from build123d import *

# Parameters (mm, degrees)
SKETCH1_R           = 1.5
SKETCH1_W           = 3
SKETCH1_H           = 7.2
SKETCH1_H_2         = 5
BOSS_EXTRUDE1_DEPTH = 3.5
FILLET1_R           = 2


with BuildPart() as part:
    # Sketch1 → Boss-Extrude1 (new body)
    with BuildSketch(Plane.XY):
        with BuildLine():
            Line((-6, 90), (-6, 5.139066063))
            ThreePointArc((-6, 5.139066063), (0, -7.9), (6, 5.139066063))
            Line((6, 5.139066063), (6, 90))
            ThreePointArc((6, 90), (0, 96), (-6, 90))
        make_face()
        Circle(SKETCH1_R, mode=Mode.SUBTRACT)
        with Locations((0, 60.876985236)):
            Circle(SKETCH1_R, mode=Mode.SUBTRACT)
        with Locations((0, 90)):
            Circle(SKETCH1_R, mode=Mode.SUBTRACT)
        with Locations((0, 25.976985236)):
            Rectangle(SKETCH1_W, SKETCH1_H, mode=Mode.SUBTRACT)
        with Locations((0, 79.876985236)):
            Rectangle(SKETCH1_W, SKETCH1_H_2, mode=Mode.SUBTRACT)
    extrude(amount=BOSS_EXTRUDE1_DEPTH)

    # Fillet1
    fillet1_edges = [part.edges().sort_by_distance(p)[0] for p in [
        (6, 5.139066063, 1.75),
        (-6, 5.139066063, 1.75),
    ]]
    fillet(fillet1_edges, radius=FILLET1_R)


solid = part.part
Design review of the part built by this model. Coordinates are the model's own, in mm. A direction names the side the tool comes from. Coordinates: 2 decimals unless noted, no trailing zeros. Write each loop counter-clockwise with the first axis right and the second up, starting at its lowest first coordinate (ties: lowest second). Pieces come first, ordered by that corner, then holes. Notation, with made-up numbers: (27.5, 74) - (55.5, 74) arc R16 ccw to (55.5, 95) - close; hole circle Ø9 at (29, -40). An arc over 180 degrees is marked (long way). Use one line per item in the form item = value.
Q1. Consider section C-C (z = 2.9). Write out the cut boundary in (x, y), plus the area to 3 significant figures.
Taken from the geometry:
outline = (-6.38, 4.65) arc R7.9 ccw (long way) to (6.38, 4.65) arc R2 cw to (6, 5.83) - (6, 90) arc R6 ccw to (-6, 90) - (-6, 5.83) arc R2 cw to start; hole circle Ø3 at (0, 0); hole (-1.5, 22.38) - (1.5, 22.38) - (1.5, 29.58) - (-1.5, 29.58) - close; hole circle Ø3 at (0, 60.88); hole (-1.5, 77.38) - (1.5, 77.38) - (1.5, 82.38) - (-1.5, 82.38) - close; hole circle Ø3 at (0, 90)
area = 1,190 mm^2
Q2. For probe 1 along Y at (x, z) = (0, 2.5); probe 2 along X at (y, z) = (90, 2.55); probe 3 along Y at (x, z) = (-1, 0.2), list the stretches that pass through material, from the lowest coordinate up.
Taken from the geometry:
probe_1 = -7.9 to -1.5, 1.5 to 22.38, 29.58 to 59.38, 62.38 to 77.38, 82.38 to 88.5, 91.5 to 96
probe_2 = -6 to -1.5, 1.5 to 6
probe_3 = -7.84 to -1.12, 1.12 to 22.38, 29.58 to 59.76, 62 to 77.38, 82.38 to 88.88, 91.12 to 95.92
Q3. Consider section B-B (x = 0). Write out the cut boundary in (y, z), plus the area to 3 significant figures.
Taken from the geometry:
outline = (-7.9, 0) - (-1.5, 0) - (-1.5, 3.5) - (-7.9, 3.5) - close; (1.5, 0) - (22.38, 0) - (22.38, 3.5) - (1.5, 3.5) - close; (29.58, 0) - (59.38, 0) - (59.38, 3.5) - (29.58, 3.5) - close; (62.38, 0) - (77.38, 0) - (77.38, 3.5) - (62.38, 3.5) - close; (82.38, 0) - (88.5, 0) - (88.5, 3.5) - (82.38, 3.5) - close; (91.5, 0) - (96, 0) - (96, 3.5) - (91.5, 3.5) - close
area = 289 mm^2
Q4. Machinability: for faces 5 (the cylindrical face through (0, 96, 2)), 6 (the flat face through (6, 47, 2)), 7 (the flat face through (0, 45, 0)), 8 (the flat face through (-6, 49, 2)), 9 (the flat face through (0, 22.377, 2)), which of the approach directions +Z, -Z, +X, -X, +Y, -Y give a long, thin tool a straight path to every point of the face, cutting with its end or side? Answer none if there is none.
Taken from the geometry:
face_5 = +Z, -Z, +Y
face_6 = +Z, -Z, +X, +Y
face_7 = -Z, +X, -X, +Y, -Y
face_8 = +Z, -Z, -X, +Y
face_9 = +Z, -Z
Q5. The part is to be moulded in two halves that separate along Y. For faces 1 (the flat face through (-1.5, 26, 2)), 2 (the cylindrical face through (-0.195, 91.487, 1.726)), 3 (the flat face through (0, 45, 3.5)), 4 (the cylindrical face through (-0.243, -7.896, 1.726)), say which applies: +Y half, -Y half, draft (parallel to the pull), parting line (faces both ways), or undercut.
Taken from the geometry:
face_1 = undercut
face_2 = undercut
face_3 = draft
face_4 = parting line
Q6. Insertion check: pin 1 Ø1.5 at (x, z) = (0.5, 1.5) entering from -Y; pin 2 Ø1 at (y, z) = (79, 1.5) entering from -X; pin 3 Ø1.5 at (x, z) = (1, 2) entering from +Y; pin 4 Ø1 at (y, z) = (55.5, 2.5) entering from +X. Each pin has a flat end and moves straight along its axis. Give the tip position at first contact, or say it passes through.
Taken from the geometry:
pin_1 = -7.9
pin_2 = -6
pin_3 = 95.99
pin_4 = 6
Q7. Consider section A-A (y = 0). Write out the cut boundary in (x, z), plus the area to 3 significant figures.
Taken from the geometry:
outline = (-7.9, 0) - (-1.5, 0) - (-1.5, 3.5) - (-7.9, 3.5) - close; (1.5, 0) - (7.9, 0) - (7.9, 3.5) - (1.5, 3.5) - close
area = 44.8 mm^2
Q8. Consider section D-D (y = 42.5). Write out the cut boundary in (x, z), plus the area to 3 significant figures.
Taken from the geometry:
outline = (-6, 0) - (6, 0) - (6, 3.5) - (-6, 3.5) - close
area = 42.0 mm^2
